Read the model definition and answer for the solid it produces. Units are mm, in the model's axes. Face numbers are marked on the shaded views. A direction names the side the tool comes from. Give positions to 0.01 mm unless a question says otherwise; leave off trailing zeros. Order: outer loops, then holes, each group sorted by start corner. A loop starts at its lowest first (then second) coordinate and runs counter-clockwise, first axis right, second up. Notation, with made-up numbers: (45, 50) -> (49, 50) arc R20 cw to (49, 68) -> close; hole circle Ø10 at (4.25, 2.5). An arc over 180 degrees is marked (long way). Use one line per item in the form item = value.
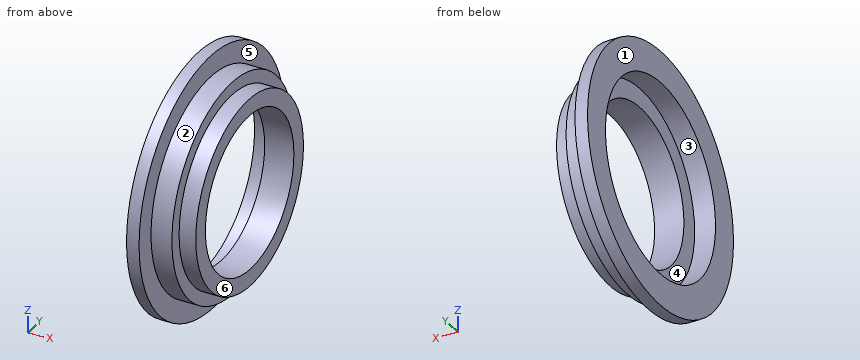
Autodesk Inventor part; units mm, degrees
ref_plane "YZ Plane" through (0, 0, 0) normal (1, 0, 0) x (0, 1, 0)
ref_plane "XZ Plane" through (0, 0, 0) normal (0, 1, 0) x (-1, 0, 0)
ref_plane "XY Plane" through (0, 0, 0) normal (0, 0, 1) x (1, 0, 0)
sketch "Sketch1" plane through (0, 0, 0) normal (0, 0, 1) x (1, 0, 0)
  line L0 (0, 0) -> (10, 0)
  line L1 (0, 23) -> (5, 23)
  line L2 (5, 23) -> (5, 18.5)
  line L3 (12, 18.5) -> (12, 22.5)
  line L4 (12, 22.5) -> (9.5, 22.5)
  line L5 (0, 30.5) -> (0, 23)
  line L6 (5, 18.5) -> (12, 18.5)
  line L7 (0, 30.5) -> (3, 30.5)
  line L8 (3, 30.5) -> (3, 25.5)
  line L9 (3, 25.5) -> (8, 25.5)
  line L10 (8, 25.5) -> (8, 22.5)
  line L11 (8, 22.5) -> (9.5, 22.5)
  dimension "d0" = 10
  dimension "d1" = 23
  dimension "d2" = 5
  dimension "d4" = 7
  dimension "d9" = 4.5
  dimension "d10" = 18.5
  dimension "d11" = 3
  dimension "d12" = 5
  dimension "d13" = 5
revolve "Revolution1" add sketch "Sketch1" angle 360 about axis through (0, 0, 0) along (1, 0, 0)
properties part number "raccord rous libre"
Item 1: Given pin 1 Ø3 at (x, y) = (10.5, -22) entering from -Z; pin 2 Ø10 at (y, z) = (17.5, 20.5) entering from -X; pin 3 Ø23 at (y, z) = (-8.5, 2.5) entering from -X; pin 4 Ø1 at (x, z) = (7, -7.5) entering from +Y, each flat-ended and moving along its own axis, determine where each tip first touches the part or whether it passes through.
Checks:
pin_1 = -9.27
pin_2 = 0
pin_3 = 5
pin_4 = 24.52
Item 2: The part is cut by section C-C on x = 6. Give the vertices of the cut face in (y, z).
Checks:
outline = circle Ø51 at (0, 0); hole circle Ø37 at (0, 0)
Item 3: Straight lines are drawn through the part: L1, parallel to Z at x = 2.55, y = 0; L2, parallel to Y at x = 8.5, z = -11; L3, parallel to Z at x = 7.5, y = 0. For each, find the intervals that lie inside material, in ascending order. Write a range as from..to.
Checks:
L1 = -30.5..-23, 23..30.5
L2 = -19.63..-14.87, 14.87..19.63
L3 = -25.5..-18.5, 18.5..25.5
Item 4: Determine the mould class of the marked faces 1, 2, 3 and 4 for opening direction Y: +Y half, -Y half, draft (parallel to the pull), parting line (faces both ways), or undercut.
Checks:
face_1 = draft
face_2 = parting line
face_3 = undercut
face_4 = undercut
Item 5: The part is cut by section A-A on z = 0. Give the vertices of the cut face in (x, y).
Checks:
outline = (0, -30.5) -> (3, -30.5) -> (3, -25.5) -> (8, -25.5) -> (8, -22.5) -> (12, -22.5) -> (12, -18.5) -> (5, -18.5) -> (5, -23) -> (0, -23) -> close; (0, 23) -> (5, 23) -> (5, 18.5) -> (12, 18.5) -> (12, 22.5) -> (8, 22.5) -> (8, 25.5) -> (3, 25.5) -> (3, 30.5) -> (0, 30.5) -> close
Item 6: The part is cut by section D-D on y = 21. Give the vertices of the cut face in (x, z).
Checks:
outline = (0, -22.12) -> (3, -22.12) -> (3, -14.47) -> (8, -14.47) -> (8, -8.08) -> (12, -8.08) -> (12, 8.08) -> (8, 8.08) -> (8, 14.47) -> (3, 14.47) -> (3, 22.12) -> (0, 22.12) -> (0, 9.38) -> (5, 9.38) -> (5, -9.38) -> (0, -9.38) -> close
Item 7: Which of the six approach directions +Z, -Z, +X, -X, +Y, -Y give full straight-line access (tool end or side, diameter ignored) to the marked faces 5 and 6?
Checks:
face_5 = +X
face_6 = +Z, -Z, +X, +Y, -Y
